Verification items for the finished model (mm, model axes). A direction names the side the tool comes from. Round coordinates to 2 decimals unless told otherwise and drop trailing zeros. Loops run counter-clockwise (first coordinate to the right, second up) from the corner with the lowest first, then second, coordinate; pieces in that order, holes last. Notation, with made-up numbers: (-33.75, 31) -> (-14.75, 31) arc R18 ccw to (-14.75, 49) -> close; hole circle Ø4 at (59.25, 56.25). An arc over 180 degrees is marked (long way). Use a Markdown table: item, result. Add a question column.
```python
from build123d import *

# Parameters (mm, degrees)
F0_R     = 107.5
F1_DEPTH = 5
F2_R     = 100
F3_DEPTH = 6
F4_R     = 102.5
F4_R_2   = 100
F5_DEPTH = 5
F6_R     = 102.5
F7_DEPTH = 5
F8_R     = 4.99999


# Not quite as in the source:
# - a fillet or chamfer is up to 0.001 mm smaller than in the source, because OpenCascade refuses the exact size


with BuildPart() as f1:
    # F0 (on Top) → F1 (new body)
    with BuildSketch(Plane.XY):
        Circle(F0_R)
    extrude(amount=F1_DEPTH)

    # F2 (on face) → F3 (cut)
    with BuildSketch(Plane.XY.offset(5)):
        Circle(F2_R)
    extrude(amount=-F3_DEPTH, mode=Mode.SUBTRACT)

    # F4 (on face) → F5 (join)
    with BuildSketch(Plane.XY.offset(5)):
        Circle(F4_R)
        Circle(F4_R_2, mode=Mode.SUBTRACT)
    extrude(amount=F5_DEPTH)

    # F6 (on face) → F7 (join)
    with BuildSketch(Plane.XY.offset(10)):
        Circle(F6_R)
    extrude(amount=F7_DEPTH)

    # F8 (radius 5 in the source; OpenCascade refuses exactly that, so slightly less here)
    f8_edges = [f1.edges().sort_by_distance(p)[0] for p in [
        (-102.5, 0, 15),
    ]]
    fillet(f8_edges, radius=F8_R)


solid = f1.part
```
1) Access from +Z, -Z, +X, -X, +Y, -Y to the whole of each face (thin tool, end or side, straight path). Record for faces 1 (the face through (95, -39, 5)), 2 (the face through (-85.31, -65.41, 2.46)).
2) Thickness scan on line 1 (Y direction, x = 0, z = 8.15); line 2 (Z direction, x = 49, y = 42.5); line 3 (Y direction, x = 0, z = 2.7). Record the ranges inside material, lowest first.
3) Sectioned sample at A-A on y = 0. Enter the section's corners in (x, z), then the cut area to 3 significant figures.
4) Sectioned sample at C-C on z = 7.5. Enter the section's corners in (x, y), then the cut area to 3 significant figures.
5) Release check for a two-part mould opening along Y. For faces 3 (the face through (-22.22, -100.063, 7.465)), 4 (the face through (-1, 1, 15)), 5 (the face through (-1, 1, 10)) record: released by +Y, released by -Y, zero draft, split by the parting line, or undercut.
6) Go/stop test with flat-tipped pins: pin 1 (6 mm diameter, centred on x = 28, z = 2.5, fed in from -Y); pin 2 (5 mm diameter, centred on y = 9, z = 9, fed in from -X); pin 3 (6 mm diameter, centred on x = 35, y = 20, fed in from -Z). Record where each tip stops, or that it passes through.
Geometry results:
| question | item | result |
|---|---|---|
| 1 | face 1 | +Z |
| 1 | face 2 | +Z, -Z |
| 2 | line 1 | -102.5 to -100, 100 to 102.5 |
| 2 | line 2 | 10 to 15 |
| 2 | line 3 | -107.5 to -100, 100 to 107.5 |
| 3 | outline | (-107.5, 0) -> (-100, 0) -> (-100, 10) -> (100, 10) -> (100, 0) -> (107.5, 0) -> (107.5, 5) -> (102.5, 5) -> (102.5, 10) arc R5 ccw to (97.5, 15) -> (-97.5, 15) arc R5 ccw to (-102.5, 10) -> (-102.5, 5) -> (-107.5, 5) -> close |
| 3 | area | 1,110 mm^2 |
| 4 | outline | circle Ø205 at (0, 0); hole circle Ø200 at (0, 0) |
| 4 | area | 1,590 mm^2 |
| 5 | face 3 | split by the parting line |
| 5 | face 4 | zero draft |
| 5 | face 5 | undercut |
| 6 | pin 1 | y = -104.55 |
| 6 | pin 2 | x = -102.29 |
| 6 | pin 3 | z = 10 |
